Read the model definition and answer for the solid it produces. Units are mm, in the model's axes. Face numbers are marked on the shaded views. A direction names the side the tool comes from. Round coordinates to 2 decimals unless told otherwise and drop trailing zeros. Write each loop counter-clockwise with the first axis right and the second up, starting at its lowest first coordinate (ties: lowest second). Pieces come first, ordered by that corner, then holes. Notation, with made-up numbers: (-14.75, 38) -> (13.25, 38) arc R22 cw to (13.25, 47) -> close; hole circle Ø6 at (-9, 8.25). An arc over 180 degrees is marked (long way). Return JSON: item names as keys, results as strings.
from build123d import *

# Parameters (mm, degrees)
F0_W     = 42
F0_H     = 42
F0_R     = 1.5
F0_R_2   = 11
F1_DEPTH = 48
F2_DEPTH = 2
F3_R     = 2.5
F4_DEPTH = 22


with BuildPart() as f1:
    # F0 (on Top) → F1 (new body)
    with BuildSketch(Plane.XY):
        Rectangle(F0_W, F0_H)
        with Locations((-15.5, -15.5)):
            Circle(F0_R, mode=Mode.SUBTRACT)
        with Locations((15.5, -15.5)):
            Circle(F0_R, mode=Mode.SUBTRACT)
        with Locations((-15.5, 15.5)):
            Circle(F0_R, mode=Mode.SUBTRACT)
        Circle(F0_R_2, mode=Mode.SUBTRACT)
        with Locations((15.5, 15.5)):
            Circle(F0_R, mode=Mode.SUBTRACT)
        Circle(F0_R_2)
    extrude(amount=-F1_DEPTH)

    # F0 (on Top) → F2 (join)
    with BuildSketch(Plane.XY):
        Circle(F0_R_2)
    extrude(amount=F2_DEPTH)

    # F3 (on face) → F4 (join)
    with BuildSketch(Plane.XY.offset(2)):
        Circle(F3_R)
    extrude(amount=F4_DEPTH)


solid = f1.part
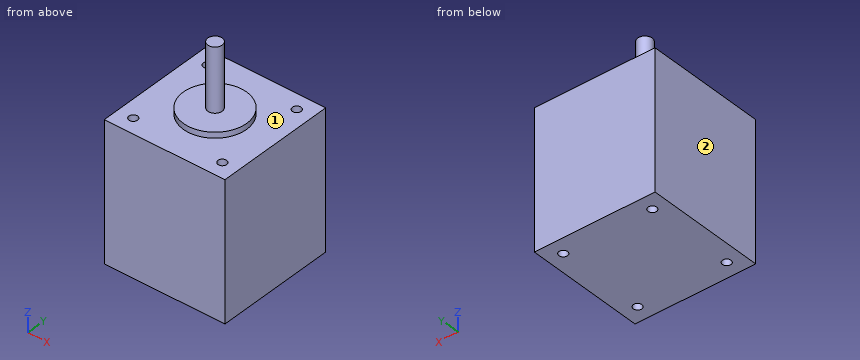
Item 1: A tool of negligible diameter and unlimited length cuts with its end or side. For the marked faces 1 and 2, from which of +Z, -Z, +X, -X, +Y, -Y can it reach the whole face along a straight path? Write none if from no direction.
Worked answers:
{"face 1": "+Z", "face 2": "+Z, -Z, -X, +Y, -Y"}
Item 2: Straight lines are drawn through the part: L1, parallel to Y at x = 15.5, z = -38; L2, parallel to X at y = -16, z = -26; L3, parallel to Z at x = -8.5, y = -16. For each, find the intervals that lie inside material, in ascending order. Write a range as [from, to].
Worked answers:
{"L1": "y = [-21, -17], [-14, 14], [17, 21]", "L2": "x = [-21, -16.91], [-14.09, 14.09], [16.91, 21]", "L3": "z = [-48, 0]"}
Item 3: Section C-C (z = -37.5) is taken. Give the vertices of the cut face in (x, y).
Worked answers:
{"outline": "(-21, -21) -> (21, -21) -> (21, 21) -> (-21, 21) -> close; hole circle Ø3 at (-15.5, -15.5); hole circle Ø3 at (-15.5, 15.5); hole circle Ø3 at (15.5, -15.5); hole circle Ø3 at (15.5, 15.5)"}
Item 4: Section A-A (y = 0) is taken. Give the vertices of the cut face in (x, z), then the cut area to 3 significant figures.
Worked answers:
{"outline": "(-21, -48) -> (21, -48) -> (21, 0) -> (11, 0) -> (11, 2) -> (2.5, 2) -> (2.5, 24) -> (-2.5, 24) -> (-2.5, 2) -> (-11, 2) -> (-11, 0) -> (-21, 0) -> close", "area": "2,170 mm2"}
Item 5: Section D-D (x = 1.5) is taken. Give the vertices of the cut face in (y, z), then the cut area to 3 significant figures.
Worked answers:
{"outline": "(-21, -48) -> (21, -48) -> (21, 0) -> (10.9, 0) -> (10.9, 2) -> (2, 2) -> (2, 24) -> (-2, 24) -> (-2, 2) -> (-10.9, 2) -> (-10.9, 0) -> (-21, 0) -> close", "area": "2,150 mm2"}
Item 6: A flat-ended cylindrical pin translates along its axis: pin 1 (5 mm diameter, centred on x = -5, y = -15, fed in from +Z). Find the tip coordinate at first contact, or state that the pin passes through.
Worked answers:
{"pin 1": "stops at z = 0"}
Item 7: Section B-B (x = 15.5) is taken. Give the vertices of the cut face in (y, z).
Worked answers:
{"outline": "(-21, -48) -> (-17, -48) -> (-17, 0) -> (-21, 0) -> close; (-14, -48) -> (14, -48) -> (14, 0) -> (-14, 0) -> close; (17, -48) -> (21, -48) -> (21, 0) -> (17, 0) -> close"}
